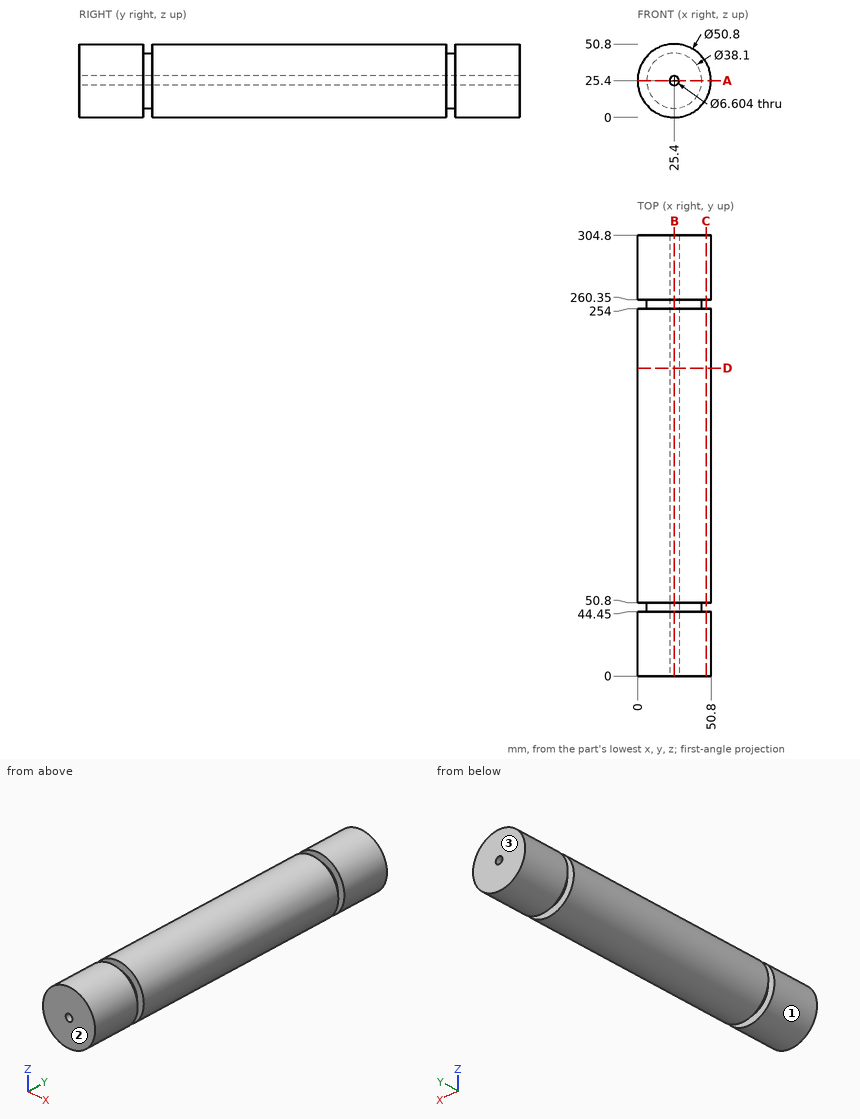
Geometry: see drawing. Coordinates: mm, zero at the bounding-box minimum. Coordinates: 2 decimals unless noted, no trailing zeros. Order: outer loops, then holes, each group sorted by start corner. A loop starts at its lowest first (then second) coordinate and runs counter-clockwise, first axis right, second up. Notation, with made-up numbers: M 48,-22 L 57,-22 A18 ccw 57,9 Z; hole C 65.25,48.25 d5. An arc over 180 degrees is marked long. Write each question's results on one line, items separated by ' | '. Start each with the question number.
1) Section query A-A (z = 25.4). Return the cut outline in (x, y), plus the area to 3 significant figures.
2) Section query D-D (y = 213). Return the cut outline in (x, z).
3) Section query C-C (x = 47.5). Return the cut outline in (y, z).
4) Draft query along Y for the marked faces 1, 2 and 3. Return one class per face: released by +Y, released by -Y, zero draft, split by the parting line, or undercut.
5) Section query B-B (x = 25.4). Return the cut outline in (y, z), plus the area to 3 significant figures.
6) Line query: line 1 (Y direction, x = 29, z = 48.5); line 2 (Z direction, x = 25.4, y = 211.5); line 3 (X direction, y = 223, z = 25). Output: solid intervals per line, ascending. Write a range as from..to.
7) Contact query for flat-ended pins moving along their axis: pin 1 Ø6 at (x, y) = (11, 125.5) entering from -Z; pin 2 Ø2 at (y, z) = (60.5, 12.5) entering from -X; pin 3 Ø5 at (x, y) = (28, 129.5) entering from -Z; pin 4 Ø4 at (x, z) = (25.4, 25.4) entering from -Y. Output: stop coordinate, or through.
Answers:
1) outline: M 0,0 L 22.1,0 L 22.1,304.8 L 0,304.8 L 0,260.35 L 6.35,260.35 L 6.35,254 L 0,254 L 0,50.8 L 6.35,50.8 L 6.35,44.45 L 0,44.45 Z; M 28.7,0 L 50.8,0 L 50.8,44.45 L 44.45,44.45 L 44.45,50.8 L 50.8,50.8 L 50.8,254 L 44.45,254 L 44.45,260.35 L 50.8,260.35 L 50.8,304.8 L 28.7,304.8 Z | area: 13,300 mm^2
2) outline: C 25.4,25.4 d50.8; hole C 25.4,25.4 d6.6
3) outline: M 0,12.88 L 44.45,12.88 L 44.45,37.92 L 0,37.92 Z; M 50.8,12.88 L 254,12.88 L 254,37.92 L 50.8,37.92 Z; M 260.35,12.88 L 304.8,12.88 L 304.8,37.92 L 260.35,37.92 Z
4) face 1: zero draft | face 2: released by -Y | face 3: released by +Y
5) outline: M 0,0 L 44.45,0 L 44.45,6.35 L 50.8,6.35 L 50.8,0 L 254,0 L 254,6.35 L 260.35,6.35 L 260.35,0 L 304.8,0 L 304.8,22.1 L 0,22.1 Z; M 0,28.7 L 304.8,28.7 L 304.8,50.8 L 260.35,50.8 L 260.35,44.45 L 254,44.45 L 254,50.8 L 50.8,50.8 L 50.8,44.45 L 44.45,44.45 L 44.45,50.8 L 0,50.8 Z | area: 13,300 mm^2
6) line 1: y = 0..44.45, 50.8..254, 260.35..304.8 | line 2: z = 0..22.1, 28.7..50.8 | line 3: x = 0..22.12, 28.68..50.8
7) pin 1: stops at z = 2.7 | pin 2: stops at x = 2.96 | pin 3: stops at z = 0 | pin 4: passes through
